from build123d import *

# Parameters (mm, degrees)
F2_W     = 17.4498
F2_H     = 13.087348
F4_DEPTH = 7.8994
F3_R     = 12.4968
F5_DEPTH = 42.9006
F1_R     = 4.953
F6_DEPTH = 50.8


with BuildPart() as f4:
    # F2 (on Front) → F4 (new body)
    with BuildSketch(Plane.XZ):
        Rectangle(F2_W, F2_H)
    extrude(amount=F4_DEPTH)

    # F3 (on offset) → F5 (join)
    with BuildSketch(Plane.XZ.offset(7.8994)):
        Circle(F3_R)
    extrude(amount=F5_DEPTH)

    # F1 (on Front) → F6 (cut)
    with BuildSketch(Plane.XZ):
        Circle(F1_R)
    extrude(amount=F6_DEPTH, mode=Mode.SUBTRACT)


solid = f4.part
Input: part model. Units: mm. Frame: model coordinates. A direction names the side the tool comes from. Give positions to 0.01 mm unless a question says otherwise; leave off trailing zeros. Write each loop counter-clockwise with the first axis right and the second up, starting at its lowest first coordinate (ties: lowest second). Pieces come first, ordered by that corner, then holes. Notation, with made-up numbers: (71.25, 64.25) -> (126.25, 64.25) arc R23 cw to (126.25, 88.25) -> close; hole circle Ø2 at (2, 32.5). An arc over 180 degrees is marked (long way). Use one line per item in the form item = value. Start each with the question number.
1) Section query A-A on x = 0. Return the cut outline in (y, z), then the cut area to 3 significant figures.
2) Section query B-B on z = 0. Return the cut outline in (x, y), then the cut area to 3 significant figures.
3) Section query D-D on x = -5.5. Return the cut outline in (y, z), then the cut area to 3 significant figures.
4) Ray query, probe 1 along Z at (x, y) = (0, -25); probe 2 along Z at (x, y) = (0.25, -45.5); probe 3 along Y at (x, z) = (-3, -8.5). Return the intervals inside material, ascending. Write a range as from..to.
5) Draft query along X for faces 4 (the cylindrical face through (11.92, -29.05, 3.75)), 5 (the cylindrical face through (-0.64, -25.04, 4.91)), 6 (the flat face through (8.725, -4, 0)). Return one class per face: pulls with the +X half, pulls with the -X half, needs draft (parallel to the pull), parting line crosses it, or undercut.
6) Set-up query: faces 1 (the flat face through (0, -4, 6.544)), 2 (the flat face through (0, -4, -6.544)), 3 (the flat face through (-8.725, -4, 0)). Return all of +Z, -Z, +X, -X, +Y, -Y with unobstructed straight access to the full face (end or side cutting, diameter ignored); none if empty.
7) Pin query (flat end, axial travel): pin 1 (10 mm diameter, centred on x = 7.5, y = -7.5, fed in from -Z); pin 2 (3 mm diameter, centred on y = -6, z = 2.5, fed in from +X); pin 3 (6 mm diameter, centred on y = -26, z = -9.5, fed in from +X). Return the tip coordinate at first contact, or that it passes through.
8) Section query C-C on y = -19.5. Return the cut outline in (x, z), then the cut area to 3 significant figures.
Outcome:
q1.outline = (-50.8, -12.5) -> (-7.9, -12.5) -> (-7.9, -6.54) -> (0, -6.54) -> (0, -4.95) -> (-50.8, -4.95) -> close; (-50.8, 4.95) -> (0, 4.95) -> (0, 6.54) -> (-7.9, 6.54) -> (-7.9, 12.5) -> (-50.8, 12.5) -> close
q1.area = 672 mm^2
q2.outline = (-12.5, -50.8) -> (-4.95, -50.8) -> (-4.95, 0) -> (-8.72, 0) -> (-8.72, -7.9) -> (-12.5, -7.9) -> close; (4.95, -50.8) -> (12.5, -50.8) -> (12.5, -7.9) -> (8.72, -7.9) -> (8.72, 0) -> (4.95, 0) -> close
q2.area = 707 mm^2
q3.outline = (-50.8, -11.22) -> (-7.9, -11.22) -> (-7.9, -6.54) -> (0, -6.54) -> (0, 6.54) -> (-7.9, 6.54) -> (-7.9, 11.22) -> (-50.8, 11.22) -> close
q3.area = 1,070 mm^2
q4.probe_1 = -12.5..-4.95, 4.95..12.5
q4.probe_2 = -12.49..-4.95, 4.95..12.49
q4.probe_3 = -50.8..-7.9
q5.face_4 = parting line crosses it
q5.face_5 = undercut
q5.face_6 = pulls with the +X half
q6.face_1 = +Z, +X, -X, +Y
q6.face_2 = -Z, +X, -X, +Y
q6.face_3 = +Z, -Z, -X, +Y
q7.pin_1 = -12.24
q7.pin_2 = 8.72
q7.pin_3 = 10.67
q8.outline = circle Ø24.99 at (0, 0); hole circle Ø9.91 at (0, 0)
q8.area = 414 mm^2
